Input: part model. Units: mm. Frame: model coordinates. A direction names the side the tool comes from. Coordinates: 2 decimals unless noted, no trailing zeros. Loops run counter-clockwise (first coordinate to the right, second up) from the corner with the lowest first, then second, coordinate; pieces in that order, holes last. Notation, with made-up numbers: (7, -29.75) - (18, -29.75) arc R14 ccw to (18, -4.75) - close; hole circle Ø5 at (44, -14.5). An arc over 180 degrees is marked (long way). Use one line per item in the form item = value.
from build123d import *

# Parameters (mm, degrees)
F1_DEPTH = 90
F3_DEPTH = 86
F5_DEPTH = 86
F7_DEPTH = 4
F9_DEPTH = 20
F10_R    = 10


with BuildPart() as f1:
    # F0 (on Front) → F1 (new body)
    with BuildSketch(Plane.XZ):
        Polygon((-22.699524987, 44.5503262094), (0, 0), (48.49, 0), (76.4529137011, 41.4496737906), (53.7533887141, 86), (5.2633887141, 86), align=None)
    extrude(amount=-F1_DEPTH)

    # F2 (on face) → F3 (cut)
    with BuildSketch(Plane(origin=(0, 90, 0), x_dir=(-1, 0, 0), z_dir=(0, 1, 0))):
        Polygon((-53.7533887141, 86), (-76.4529137011, 41.4496737906), (22.699524987, 44.5503262094), (-5.2633887141, 86), align=None)
    extrude(amount=-F3_DEPTH, mode=Mode.SUBTRACT)

    # F4 (on face) → F5 (cut)
    with BuildSketch(Plane(origin=(0, 90, 0), x_dir=(-1, 0, 0), z_dir=(0, 1, 0))):
        Polygon((-74.4529137011, 41.5122169304), (-47.7970534464, 2), (-0.9490817796, 2), (20.699524987, 44.4877830696), align=None)
    extrude(amount=-F5_DEPTH, mode=Mode.SUBTRACT)

    # F6 (on face) → F7 (join)
    with BuildSketch(Plane(origin=(0, 90, 0), x_dir=(-1, 0, 0), z_dir=(0, 1, 0))):
        Polygon((22.699524987, 44.5503262094), (-76.4529137011, 41.4496737906), (-48.49, 0), (0, 0), align=None)
    extrude(amount=-F7_DEPTH)

    # F8 (on face) → F9 (join)
    with BuildSketch(Plane.XZ):
        with BuildLine():
            Line((41.8766943571, 28), (41.8766943571, 43))
            ThreePointArc((41.8766943571, 43), (37.4832960749, 32.3933982822), (26.8766943571, 28))
            Line((26.8766943571, 28), (41.8766943571, 28))
        make_face()
        with BuildLine():
            ThreePointArc((26.8766943571, 58), (37.4832960749, 53.6066017178), (41.8766943571, 43))
            Line((41.8766943571, 43), (41.8766943571, 58))
            Line((41.8766943571, 58), (26.8766943571, 58))
        make_face()
        with BuildLine():
            ThreePointArc((11.8766943571, 43), (16.2700926393, 53.6066017178), (26.8766943571, 58))
            Line((26.8766943571, 58), (11.8766943571, 58))
            Line((11.8766943571, 58), (11.8766943571, 43))
        make_face()
        with BuildLine():
            ThreePointArc((26.8766943571, 28), (37.4832960749, 32.3933982822), (41.8766943571, 43))
            ThreePointArc((41.8766943571, 43), (37.4832960749, 53.6066017178), (26.8766943571, 58))
            ThreePointArc((26.8766943571, 58), (16.2700926393, 53.6066017178), (11.8766943571, 43))
            ThreePointArc((11.8766943571, 43), (16.2700926393, 32.3933982822), (26.8766943571, 28))
        make_face()
        with BuildLine():
            Line((11.8766943571, 28), (26.8766943571, 28))
            ThreePointArc((26.8766943571, 28), (16.2700926393, 32.3933982822), (11.8766943571, 43))
            Line((11.8766943571, 43), (11.8766943571, 28))
        make_face()
    extrude(amount=F9_DEPTH)

    # F10
    f10_edges = [f1.edges().sort_by_distance(p)[0] for p in [
        (11.876694, -10, 58),
        (41.876694, -10, 58),
        (11.876694, -10, 28),
        (41.876694, -10, 28),
    ]]
    fillet(f10_edges, radius=F10_R)


solid = f1.part
Q1. Cut plane D-D, the plane z = 9.5. Return loops of the section in (x, y).
Check values:
outline = (-4.84, 0) - (54.9, 0) - (54.9, 90) - (-4.84, 90) - close; hole (-2.87, 4) - (52.86, 4) - (52.86, 86) - (-2.87, 86) - close
Q2. Pull-direction query (X, two-part tool) for faces 6 (the flat face through (-9.7, 45.6, 22.9)), 7 (the flat face through (62.276, 44.37, 20.435)), 8 (the flat face through (26, 90, 23)); classes: pulls with the +X half, pulls with the -X half, needs draft (parallel to the pull), parting line crosses it, or undercut.
Check values:
face_6 = undercut
face_7 = pulls with the +X half
face_8 = needs draft
Q3. Cut plane B-B, the plane z = 30.5. Return loops of the section in (x, y), then the cut area to 3 significant figures.
Check values:
outline = (-15.54, 0) - (15.26, 0) - (15.26, -20) - (38.49, -20) - (38.49, 0) - (69.07, 0) - (69.07, 90) - (-15.54, 90) - close; hole (-13.57, 4) - (67.02, 4) - (67.02, 86) - (-13.57, 86) - close
area = 1,470 mm²
Q4. Ray query, line 1 along Z through (x, y) = (33, 73.5); line 2 along Y through (x, z) = (43, 79.5); line 3 along Y through (x, z) = (30.5, 50). Return the intervals inside material, ascending. Write a range as [from, to].
Check values:
line_1 = [0, 2]
line_2 = [0, 4]
line_3 = [-20, 4]
Q5. Cut plane A-A, the plane y = -3. Return loops of the section in (x, z).
Check values:
outline = (11.88, 38) arc R10 ccw to (21.88, 28) - (31.88, 28) arc R10 ccw to (41.88, 38) - (41.88, 48) arc R10 ccw to (31.88, 58) - (21.88, 58) arc R10 ccw to (11.88, 48) - close
Q6. Set-up query: faces 1 (the cylindrical face through (39.03, -10.14, 54.99)), 2 (the flat face through (27, -10, 28)), 3 (the cylindrical face through (39.03, -10.14, 31.01)), 4 (the flat face through (41.877, -10, 43)), 5 (the flat face through (27, -10, 58)). Return all of +Z, -Z, +X, -X, +Y, -Y with unobstructed straight access to the full face (end or side cutting, diameter ignored); none if empty.
Check values:
face_1 = +Z, +X, -Y
face_2 = -Z, +X, -X, -Y
face_3 = -Z, +X, -Y
face_4 = +Z, -Z, +X, -Y
face_5 = +Z, +X, -X, -Y
Q7. Cut plane C-C, the plane x = 63.5. Return loops of the section in (y, z).
Check values:
outline = (0, 22.25) - (90, 22.25) - (90, 41.85) - (86, 41.85) - (86, 25.28) - (4, 25.28) - (4, 66.87) - (0, 66.87) - close
Q8. First-contact query: P1, Ø3, axis at x = 20, z = 74, coming from the -Y side; P2, Ø8, axis at y = -7, z = 40.5, coming from the +X side; P3, Ø11, axis at y = -9, z = 45.5, coming from the -X side. Flat tips, straight axial feed; report the tip coordinate or a pass-through.
Check values:
P1 = 0
P2 = 41.88
P3 = 11.88
